Autodesk Inventor part; units mm, degrees
ref_plane "YZ Plane" through (0, 0, 0) normal (1, 0, 0) x (0, 1, 0)
ref_plane "XZ Plane" through (0, 0, 0) normal (0, 1, 0) x (-1, 0, 0)
ref_plane "XY Plane" through (0, 0, 0) normal (0, 0, 1) x (1, 0, 0)
sketch "Sketch1" plane through (0, 0, 0) normal (0, 0, 1) x (1, 0, 0)
  circle A0 centre (0, 0) radius 4.1275
  line L0 (-6.35, 6.35) -> (6.35, 6.35)
  line L1 (6.35, 6.35) -> (6.35, -4.2672)
  line L2 (6.35, -4.2672) -> (-6.35, -4.2672)
  line L3 (-6.35, -4.2672) -> (-6.35, 6.35)
  line L4 (-3.175, -4.2672) -> (3.175, -4.2672)
  line L5 (3.175, -4.2672) -> (3.175, -7.4422)
  line L6 (3.175, -7.4422) -> (-3.175, -7.4422)
  line L7 (-3.175, -7.4422) -> (-3.175, -4.2672)
  dimension "d0" = 8.255
  dimension "d1" = 4.2672
  dimension "d2" = 6.35
  dimension "d3" = 6.35
  dimension "d4" = 6.35
  dimension "d5" = 3.175
  dimension "d6" = 3.175
  dimension "d7" = 3.175
extrude "Extrusion1" add sketch "Sketch1" along normal blind 3.175
properties part number "rod holder"
Model file for the job. Use its own axes, mm. A direction names the side the tool comes from. Round coordinates to 2 decimals unless told otherwise and drop trailing zeros. Loops run counter-clockwise (first coordinate to the right, second up) from the corner with the lowest first, then second, coordinate; pieces in that order, holes last.
1. Tool access for faces 5 (the flat face through (0, -7.442, 2)), 6 (the flat face through (-5, -4.267, 2)): list every direction of +Z, -Z, +X, -X, +Y, -Y with a clear straight run to the whole face (end or side of a thin tool).
Check values:
face 5: +Z, -Z, +X, -X, -Y
face 6: +Z, -Z, -X, -Y
2. Band-saw the part on D-D, the plane x = -5.5. List the corners of the cut face in (y, z) (3 decimals).
Check values:
outline: (-4.267, 0) - (6.35, 0) - (6.35, 3.175) - (-4.267, 3.175) - close
3. Mould opens along Y. For faces 1 (the cylindrical face through (3.937, -1.24, 1.565)), 2 (the flat face through (0, 6.35, 2)), 3 (the flat face through (3.175, -6, 2)), 4 (the flat face through (5, -4.267, 2)) say: +Y half, -Y half, draft (parallel to the pull), parting line (faces both ways), or undercut.
Check values:
face 1: undercut
face 2: +Y half
face 3: draft
face 4: -Y half
4. Wall check: probe 1 along Y at (x, z) = (0, 2.55); probe 2 along Y at (x, z) = (-5.25, 1.4); probe 3 along X at (y, z) = (-1.5, 2.3). Give the ranges that are in metal, low to high.
Check values:
probe 1: y = -7.44 to -4.13, 4.13 to 6.35
probe 2: y = -4.27 to 6.35
probe 3: x = -6.35 to -3.85, 3.85 to 6.35
5. Drop flat-ended pins along their axis: P1, Ø1, axis at x = -5.5, z = 2, coming from the -Y side; P2, Ø1, axis at y = -5.5, z = 1, coming from the +X side (3 decimals); P3, Ø7.5, axis at x = 0, y = 0, coming from the +Z side; P4, Ø1, axis at y = -5, z = 2, coming from the -X side (3 decimals). Give the stop position or say it passes through.
Check values:
P1: stops at y = -4.27
P2: stops at x = 3.175
P3: passes through
P4: stops at x = -3.175
